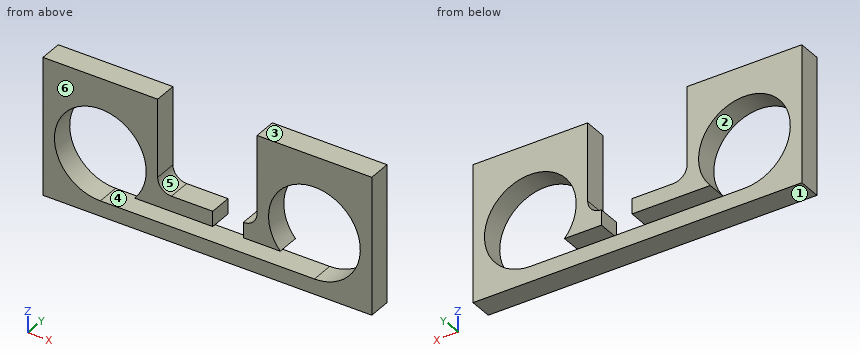
from build123d import *

# Parameters (mm, degrees)
F0_W     = 273.05
F0_H     = 114.3
F1_DEPTH = 19.05
F2_R     = 38.1
F3_DEPTH = 25.4
F5_DEPTH = 25.4
F7_DEPTH = 25.4


with BuildPart() as f1:
    # F0 (on Front) → F1 (new body)
    with BuildSketch(Plane.XZ):
        with Locations((136.525, 57.15)):
            Rectangle(F0_W, F0_H)
    extrude(amount=F1_DEPTH)

    # F2 (on face) → F3 (cut)
    with BuildSketch(Plane.XZ.offset(19.05)):
        with Locations((47.625, 50.8)):
            Circle(F2_R)
        with Locations((225.425, 50.8)):
            Circle(F2_R)
    extrude(amount=-F3_DEPTH, mode=Mode.SUBTRACT)

    # F4 (on face) → F5 (cut)
    with BuildSketch(Plane.XZ.offset(19.05)):
        with BuildLine():
            Line((177.8, 114.3), (95.25, 114.3))
            Line((95.25, 114.3), (95.25, 49.53))
            ThreePointArc((95.25, 49.53), (98.597769491, 41.447769491), (106.68, 38.1))
            Line((106.68, 38.1), (166.37, 38.1))
            ThreePointArc((166.37, 38.1), (174.452230509, 41.447769491), (177.8, 49.53))
            Line((177.8, 49.53), (177.8, 114.3))
        make_face()
    extrude(amount=-F5_DEPTH, mode=Mode.SUBTRACT)

    # F6 (on face) → F7 (cut)
    with BuildSketch(Plane.XZ.offset(19.05)):
        with BuildLine():
            Line((166.37, 38.1), (140.97, 38.1))
            Line((140.97, 38.1), (140.97, 25.4))
            Line((140.97, 25.4), (76.0230633142, 25.4))
            ThreePointArc((76.0230633142, 25.4), (63.1792598667, 16.0196175984), (47.625, 12.7))
            Line((47.625, 12.7), (225.425, 12.7))
            ThreePointArc((225.425, 12.7), (209.8707401333, 16.0196175984), (197.0269366858, 25.4))
            Line((197.0269366858, 25.4), (166.37, 25.4))
            Line((166.37, 25.4), (166.37, 38.1))
        make_face()
    extrude(amount=-F7_DEPTH, mode=Mode.SUBTRACT)


solid = f1.part
Can you work these out from the model? Positions are in its coordinate system, mm. Face numbers are marked on the shaded views. A direction names the side the tool comes from. Give positions to 0.01 mm unless a question says otherwise; leave off trailing zeros. Write each loop counter-clockwise with the first axis right and the second up, starting at its lowest first coordinate (ties: lowest second). Pieces come first, ordered by that corner, then holes. Notation, with made-up numbers: (-12, 33.5) -> (11, 33.5) arc R16 cw to (11, 37.5) -> close; hole circle Ø6 at (-16.75, 72). An arc over 180 degrees is marked (long way). Answer as a JSON object with one key per item and string values. Group by question number.
Item 1: For the marked faces 4, 5 and 6, which set-ups out of +Z, -Z, +X, -X, +Y, -Y let a thin tool reach every point of the face, with its end or its side?
Item 2: We'd pull the mould along Z, two halves only. Please class the marked faces 1, 2 and 3: +Z half, -Z half, draft (parallel to the pull), parting line (faces both ways), or undercut.
Item 3: Please list where these lines run through material, in increasing order: line 1 (X direction, y = -8.5, z = 50.8) (3 decimals); line 2 (X direction, y = -13.25, z = 91); line 3 (X direction, y = -5.5, z = 79). Write a range as [from, to].
Item 4: Suppose I cut it at D-D (y = -9.25). Please give me the cut outline in (x, z) (3 decimals).
Item 5: Suppose I cut it at A-A (x = 134). Please give me the cut outline in (y, z), plus the area to 3 significant figures.
Item 6: I'm going to push a flat-ended pin straight in: P1, Ø9.5, axis at x = 133.5, y = -12, coming from the +Z side. Where does the tip first touch, or does it pass through?
Item 7: Suppose I cut it at B-B (z = 106.5). Please give me the cut outline in (x, y), plus the area to 3 significant figures.
Item 8: Suppose I cut it at C-C (z = 57.5). Please give me the cut outline in (x, y).
Findings:
{
 "1": {"face 4": "+Y, -Y", "face 5": "+Z, +Y, -Y", "face 6": "+Z, -Z, +X, -X, -Y"},
 "2": {"face 1": "-Z half", "face 2": "undercut", "face 3": "+Z half"},
 "3": {"line 1": "x = [0, 9.525], [85.725, 95.25], [177.8, 187.325], [263.525, 273.05]", "line 2": "x = [0, 95.25], [177.8, 273.05]", "line 3": "x = [0, 22.01], [73.24, 95.25], [177.8, 199.81], [251.04, 273.05]"},
 "4": {"outline": "(0, 0) -> (273.05, 0) -> (273.05, 114.3) -> (177.8, 114.3) -> (177.8, 49.53) arc R11.43 cw to (166.37, 38.1) -> (166.37, 25.4) -> (197.027, 25.4) arc R38.1 cw (long way) to (225.425, 12.7) -> (47.625, 12.7) arc R38.1 cw (long way) to (76.023, 25.4) -> (140.97, 25.4) -> (140.97, 38.1) -> (106.68, 38.1) arc R11.43 cw to (95.25, 49.53) -> (95.25, 114.3) -> (0, 114.3) -> close"},
 "5": {"outline": "(-19.05, 0) -> (0, 0) -> (0, 12.7) -> (-19.05, 12.7) -> close; (-19.05, 25.4) -> (0, 25.4) -> (0, 38.1) -> (-19.05, 38.1) -> close", "area": "484 mm²"},
 "6": {"P1": "stops at z = 38.1"},
 "7": {"outline": "(0, -19.05) -> (95.25, -19.05) -> (95.25, 0) -> (0, 0) -> close; (177.8, -19.05) -> (273.05, -19.05) -> (273.05, 0) -> (177.8, 0) -> close", "area": "3,630 mm²"},
 "8": {"outline": "(0, -19.05) -> (10.12, -19.05) -> (10.12, 0) -> (0, 0) -> close; (85.13, -19.05) -> (95.25, -19.05) -> (95.25, 0) -> (85.13, 0) -> close; (177.8, -19.05) -> (187.92, -19.05) -> (187.92, 0) -> (177.8, 0) -> close; (262.93, -19.05) -> (273.05, -19.05) -> (273.05, 0) -> (262.93, 0) -> close"}
}
